from build123d import *

# Parameters (mm, degrees)
F0_R     = 29.709724
F1_DEPTH = 12.7
F2_R     = 51.174274
F2_R_2   = 35.519293
F3_DEPTH = 38.1
F4_R     = 35.519293
F5_DEPTH = 79.248
F6_W     = 55.42592
F6_H     = 20.859219
F7_DEPTH = 42.926
F9_DEPTH = 25.4


with BuildPart() as f1:
    # F0 (on Top) → F1 (new body)
    with BuildSketch(Plane.XY):
        with BuildLine():
            ThreePointArc((33.761899, -41.666997), (86.906989, -45.492746), (114.645897, 0))
            ThreePointArc((114.645897, 0), (86.906989, 45.492746), (33.761899, 41.666997))
            ThreePointArc((33.761899, 41.666997), (12.297348, 0), (33.761899, -41.666997))
        make_face()
        with Locations((63.471623, 0)):
            Circle(F0_R, mode=Mode.SUBTRACT)
        with BuildLine():
            ThreePointArc((33.761899, -41.666997), (12.297348, 0), (33.761899, 41.666997))
            Line((33.761899, 41.666997), (-49.168151, 41.666997))
            Line((-49.168151, 41.666997), (-49.168151, -41.666997))
            Line((-49.168151, -41.666997), (33.761899, -41.666997))
        make_face()
    extrude(amount=F1_DEPTH)

    # F2 (on face) → F3 (join)
    with BuildSketch(Plane.XY.offset(12.7)):
        with Locations((63.471623, 0)):
            Circle(F2_R)
        with Locations((63.471623, 0)):
            Circle(F2_R_2, mode=Mode.SUBTRACT)
    extrude(amount=F3_DEPTH)

    # F4 (on face) → F5 (cut)
    with BuildSketch(Plane.XY.offset(50.8)):
        with Locations((63.471623, 0)):
            Circle(F4_R)
    extrude(amount=-F5_DEPTH, mode=Mode.SUBTRACT)

    # F6 (on face) → F7 (join)
    with BuildSketch(Plane.XY.offset(12.7)):
        with Locations((-11.171911, 0.148995)):
            Rectangle(F6_W, F6_H)
    extrude(amount=F7_DEPTH)

    # F8 (on face) → F9 (cut)
    with BuildSketch(Plane.XZ.offset(10.280615)):
        Polygon((-38.884871, 70.77235), (-38.884871, 12.7), (13.340641, 50.8), (16.541049, 50.8), (16.541049, 70.77235), align=None)
    extrude(amount=-F9_DEPTH, mode=Mode.SUBTRACT)


solid = f1.part
Work out the finished part from the listing and answer in its coordinate system (mm). A direction names the side the tool comes from. Round coordinates to 2 decimals unless told otherwise and drop trailing zeros. Write each loop counter-clockwise with the first axis right and the second up, starting at its lowest first coordinate (ties: lowest second). Pieces come first, ordered by that corner, then holes. Notation, with made-up numbers: (34.25, 65) - (68.25, 65) arc R6 cw to (68.25, 75) - close; hole circle Ø11 at (-28.75, 32). An arc over 180 degrees is marked (long way). Answer in a Markdown table with one row per item. Add a question column.
1. A cutting plane is placed at D-D, the plane y = -18. Determine the outline of the cut face in (x, z), and give its area (3 significant figures).
2. A cutting plane is placed at A-A, the plane y = 21. Determine the outline of the cut face in (x, z), and give its area (3 significant figures).
3. The mould has two halves that part along X. Classify faces 5 (the flat face through (-13.14, 0, 31.48)), 6 (the flat face through (29.5, 12.1, 50.8)), 7 (the cylindrical face through (27.987, 1.562, 25.756)): +X half, -X half, draft (parallel to the pull), parting line (faces both ways), or undercut.
4. A cutting plane is placed at C-C, the plane x = 56.5. Determine the outline of the cut face in (y, z), and give its area (3 significant figures).
5. Find the intervals of material crossed by line 1 along Y through (x, z) = (64.5, 13.5); line 2 along Y through (x, z) = (-12.5, 20.5); line 3 along X through (y, z) = (13.5, 4.5), in increasing order. Write a range as from..to.
6. A cutting plane is placed at B-B, the plane z = 4.5. Determine the outline of the cut face in (x, y).
7. Given pin 1 (19 mm diameter, centred on x = -3, z = 24.5, fed in from +Y); pin 2 (3 mm diameter, centred on x = 14.5, z = 40.5, fed in from -Y); pin 3 (8 mm diameter, centred on x = -1, y = 19.5, fed in from +Z); pin 4 (5 mm diameter, centred on x = -26, y = 38, fed in from -Z), each flat-ended and moving along its own axis, determine where each tip first touches the part or whether it passes through.
8. For faces 1 (the flat face through (-2, -10.281, 27)), 2 (the flat face through (-8, -41.667, 6)), 3 (the flat face through (-7, 10.579, 27)), 4 (the flat face through (-17, 19, 12.7)), determine the directions among +Z, -Z, +X, -X, +Y, -Y from which every point of the face is accessible in a straight line to the end or side of a thin tool.
Worked out:
| question | item | result |
|---|---|---|
| 1 | outline | (-49.17, 0) - (32.85, 0) - (32.85, 50.8) - (15.57, 50.8) - (15.57, 12.7) - (-49.17, 12.7) - close; (94.09, 0) - (111.38, 0) - (111.38, 50.8) - (94.09, 50.8) - close |
| 1 | area | 2,580 mm^2 |
| 2 | outline | (-49.17, 0) - (34.83, 0) - (34.83, 50.8) - (16.8, 50.8) - (16.8, 12.7) - (-49.17, 12.7) - close; (92.12, 0) - (110.14, 0) - (110.14, 50.8) - (92.12, 50.8) - close |
| 2 | area | 2,670 mm^2 |
| 3 | face 5 | -X half |
| 3 | face 6 | draft |
| 3 | face 7 | undercut |
| 4 | outline | (-50.7, 0) - (-34.83, 0) - (-34.83, 50.8) - (-50.7, 50.8) - close; (34.83, 0) - (50.7, 0) - (50.7, 50.8) - (34.83, 50.8) - close |
| 4 | area | 1,610 mm^2 |
| 5 | line 1 | -51.16..-35.5, 35.5..51.16 |
| 5 | line 2 | -10.28..10.58 |
| 5 | line 3 | -49.17..30.62, 96.33..112.83 |
| 6 | outline | (-49.17, -41.67) - (33.76, -41.67) arc R51.17 ccw (long way) to (33.76, 41.67) - (-49.17, 41.67) - close; hole circle Ø71.04 at (63.47, 0) |
| 7 | pin 1 | y = 10.58 |
| 7 | pin 2 | y = -19.11 |
| 7 | pin 3 | z = 12.7 |
| 7 | pin 4 | z = 0 |
| 8 | face 1 | +Z, -X, -Y |
| 8 | face 2 | +Z, -Z, -X, -Y |
| 8 | face 3 | +Z, -X, +Y |
| 8 | face 4 | +Z, -X |
